For this review, take the finished solid that the model builds, in its own axes (mm). Face numbers are marked on the shaded views. A direction names the side the tool comes from. Round coordinates to 2 decimals unless told otherwise and drop trailing zeros. Write each loop counter-clockwise with the first axis right and the second up, starting at its lowest first coordinate (ties: lowest second). Pieces come first, ordered by that corner, then holes. Notation, with made-up numbers: (3, 27.25) - (55, 27.25) arc R25 ccw to (55, 55.25) - close; hole circle Ø1 at (22, 12). An arc over 180 degrees is marked (long way). One line per item, written item: value. Start each with the question number.
Q1. Mouldability with a two-part tool opening along X and no side actions: class the marked faces 1, 2 and 3 as +X half, -X half, draft (parallel to the pull), parting line (faces both ways), or undercut.
Q2. Clearance check with flat-ended pins moving along their axes: pin 1 Ø1.7 at (x, y) = (-35, -6.5) entering from +Z; pin 2 Ø1.5 at (x, z) = (18.5, 5) entering from +Y; pin 3 Ø3.5 at (x, y) = (14.75, 5) entering from -Z; pin 4 Ø3 at (y, z) = (2.5, 4) entering from +X. State where each tip first meets the part, or that it passes through.
Q3. Add section B-B on x = -9. Write out the cut boundary in (y, z).
Q4. Add section A-A on y = 0. Write out the cut boundary in (x, z).
Q5. For probe 1 along Y at (x, z) = (14.75, 1.95); probe 2 along Y at (x, z) = (-34.75, 1.75); probe 3 along X at (y, z) = (7.5, 5.5), list the stretches that pass through material, from the lowest coordinate up.
Q6. Add section C-C on x = 35. Write out the cut boundary in (y, z), and give its area (3 significant figures).
Q7. Tool access review of the marked faces 4, 5 and 6: name each direction out of +Z, -Z, +X, -X, +Y, -Y from which nothing blocks a thin tool from reaching the whole face with its end or side.
```python
from build123d import *

# Parameters (mm, degrees)
SZKIC1_R                    = 1.55
SZKIC1_R_2                  = 1.45
DODANIE_WYCI_GNI_CIE1_DEPTH = 8
WYTNIJ_WYCI_GNI_CIE1_DEPTH  = 3
ZAOKR_GLENIE1_R             = 4
WYTNIJ_WYCI_GNI_CIE2_DEPTH  = 3.5
SFAZOWANIE1_SIZE            = 0.25
WYTNIJ_WYCI_GNI_CIE3_DEPTH  = 1
WYTNIJ_WYCI_GNI_CIE4_DEPTH  = 3
SZYK_LINIOWY1_COUNT         = 2
SZYK_LINIOWY1_PITCH         = 15


with BuildPart() as part:
    # Szkic1 → Dodanie-wyciągnięcie1 (new body)
    # profile 1 of 17: a face of its own
    with BuildSketch(Plane.XY):
        with BuildLine():
            Line((-30, -5), (-30, 5))
            ThreePointArc((-30, 5), (-34.75, 9.75), (-39.5, 5))
            Line((-39.5, 5), (-39.5, -5))
            ThreePointArc((-39.5, -5), (-34.75, -9.75), (-30, -5))
        make_face()
        with Locations((-34.75, -5)):
            Circle(SZKIC1_R, mode=Mode.SUBTRACT)
        with Locations((-34.75, 5)):
            Circle(SZKIC1_R, mode=Mode.SUBTRACT)
    # profile 2 of 17: a face of its own
    with BuildSketch(Plane.XY):
        with BuildLine():
            Line((-30, -10), (-30, -5))
            ThreePointArc((-30, -5), (-34.75, -9.75), (-39.5, -5))
            ThreePointArc((-39.5, -5), (-36.846817098, -13.293438899), (-29.872582883, -18.506937282))
            ThreePointArc((-29.872582883, -18.506937282), (-32.348896474, -13.420890585), (-27.262849777, -10.944576994))
            Line((-27.262849777, -10.944576994), (-30, -10))
        make_face()
    # profile 3 of 17: a face of its own
    with BuildSketch(Plane.XY):
        with BuildLine():
            Line((4.547807332, -21.922277315), (-27.262849777, -10.944576994))
            ThreePointArc((-27.262849777, -10.944576994), (-32.348896474, -13.420890585), (-29.872582883, -18.506937282))
            Line((-29.872582883, -18.506937282), (5.695133447, -30.781180144))
            ThreePointArc((5.695133447, -30.781180144), (3.398037408, -28.739501506), (3.227247846, -25.670962309))
            Line((3.227247846, -25.670962309), (4.547807332, -21.922277315))
        make_face()
    # profile 4 of 17: a face of its own
    with BuildSketch(Plane.XY):
        with BuildLine():
            Line((7.670780796, -23), (4.547807332, -21.922277315))
            Line((4.547807332, -21.922277315), (3.227247846, -25.670962309))
            ThreePointArc((3.227247846, -25.670962309), (4.688739604, -23.735329208), (7, -23))
            Line((7, -23), (7.670780796, -23))
        make_face()
    # profile 5 of 17: a face of its own
    with BuildSketch(Plane.XY):
        with BuildLine():
            Line((10, -6.445085227), (4.547807332, -21.922277315))
            Line((4.547807332, -21.922277315), (7.670780796, -23))
            Line((7.670780796, -23), (12.650026795, -23))
            Line((12.650026795, -23), (16.842670109, -11.098302851))
            Line((16.842670109, -11.098302851), (14.743601006, -9.74999569))
            ThreePointArc((14.743601006, -9.74999569), (11.798045524, -8.721352546), (10.126086359, -6.087162658))
            Line((10.126086359, -6.087162658), (10, -6.445085227))
        make_face()
    # profile 6 of 17: a face of its own
    with BuildSketch(Plane.XY):
        with BuildLine():
            ThreePointArc((3.227247846, -25.670962309), (3.398037408, -28.739501506), (5.695133447, -30.781180144))
            ThreePointArc((5.695133447, -30.781180144), (6.338456568, -30.944915752), (7, -31))
            ThreePointArc((7, -31), (9.311260396, -30.264670792), (10.772752154, -28.329037691))
            ThreePointArc((10.772752154, -28.329037691), (10.601962592, -25.260498494), (8.304866553, -23.218819856))
            Line((8.304866553, -23.218819856), (7.670780796, -23))
            Line((7.670780796, -23), (7, -23))
            ThreePointArc((7, -23), (4.688739604, -23.735329208), (3.227247846, -25.670962309))
        make_face()
        with Locations((7, -27)):
            Circle(SZKIC1_R_2, mode=Mode.SUBTRACT)
    # profile 7 of 17: a face of its own
    with BuildSketch(Plane.XY):
        with BuildLine():
            Line((10, -5), (10, -6.445085227))
            Line((10, -6.445085227), (10.126086359, -6.087162658))
            ThreePointArc((10.126086359, -6.087162658), (10.03162688, -5.547224911), (10, -5))
        make_face()
    # profile 8 of 17: a face of its own
    with BuildSketch(Plane.XY):
        with BuildLine():
            Line((12.650026795, -23), (7.670780796, -23))
            Line((7.670780796, -23), (8.304866553, -23.218819856))
            ThreePointArc((8.304866553, -23.218819856), (10.601962592, -25.260498494), (10.772752154, -28.329037691))
            Line((10.772752154, -28.329037691), (12.650026795, -23))
        make_face()
    # profile 9 of 17: a face of its own
    with BuildSketch(Plane.XY):
        with BuildLine():
            ThreePointArc((10.772752154, -28.329037691), (9.311260396, -30.264670792), (7, -31))
            Line((7, -31), (49, -31))
            ThreePointArc((49, -31), (47.873511508, -30.838101572), (46.838211374, -30.365511839))
            Line((46.838211374, -30.365511839), (35.371448625, -23))
            Line((35.371448625, -23), (12.650026795, -23))
            Line((12.650026795, -23), (10.772752154, -28.329037691))
        make_face()
    # profile 10 of 17: a face of its own
    with BuildSketch(Plane.XY):
        with BuildLine():
            ThreePointArc((10, -5), (10.03162688, -5.547224911), (10.126086359, -6.087162658))
            Line((10.126086359, -6.087162658), (10.977247846, -3.670962309))
            ThreePointArc((10.977247846, -3.670962309), (13.45169048, -1.216563415), (16.911788626, -1.634488161))
            Line((16.911788626, -1.634488161), (19.5, -3.296988898))
            Line((19.5, -3.296988898), (19.5, 5))
            ThreePointArc((19.5, 5), (14.75, 9.75), (10, 5))
            Line((10, 5), (10, -5))
        make_face()
        with Locations((14.75, 5)):
            Circle(SZKIC1_R, mode=Mode.SUBTRACT)
    # profile 11 of 17: a face of its own
    with BuildSketch(Plane.XY):
        with BuildLine():
            Line((10.977247846, -3.670962309), (10.126086359, -6.087162658))
            ThreePointArc((10.126086359, -6.087162658), (11.798045524, -8.721352546), (14.743601006, -9.74999569))
            Line((14.743601006, -9.74999569), (12.588211374, -8.365511839))
            ThreePointArc((12.588211374, -8.365511839), (10.966563415, -6.29830952), (10.977247846, -3.670962309))
        make_face()
    # profile 12 of 17: a face of its own
    with BuildSketch(Plane.XY):
        Polygon((16.842670109, -11.098302851), (12.650026795, -23), (35.371448625, -23), align=None)
    # profile 13 of 17: a face of its own
    with BuildSketch(Plane.XY):
        with BuildLine():
            ThreePointArc((46.838211374, -30.365511839), (47.873511508, -30.838101572), (49, -31))
            ThreePointArc((49, -31), (52.838101572, -28.126488492), (51.161788626, -23.634488161))
            ThreePointArc((51.161788626, -23.634488161), (50.126488492, -23.161898428), (49, -23))
            Line((49, -23), (35.371448625, -23))
            Line((35.371448625, -23), (46.838211374, -30.365511839))
        make_face()
        with Locations((49, -27)):
            Circle(SZKIC1_R_2, mode=Mode.SUBTRACT)
    # profile 14 of 17: a face of its own
    with BuildSketch(Plane.XY):
        with BuildLine():
            ThreePointArc((16.911788626, -1.634488161), (13.45169048, -1.216563415), (10.977247846, -3.670962309))
            ThreePointArc((10.977247846, -3.670962309), (10.966563415, -6.29830952), (12.588211374, -8.365511839))
            Line((12.588211374, -8.365511839), (14.743601006, -9.74999569))
            ThreePointArc((14.743601006, -9.74999569), (16.291742556, -9.492830944), (17.671590668, -8.745238039))
            Line((17.671590668, -8.745238039), (18.522752154, -6.329037691))
            ThreePointArc((18.522752154, -6.329037691), (18.533436585, -3.70169048), (16.911788626, -1.634488161))
        make_face()
        with Locations((14.75, -5)):
            Circle(SZKIC1_R, mode=Mode.SUBTRACT)
    # profile 15 of 17: a face of its own
    with BuildSketch(Plane.XY):
        with BuildLine():
            ThreePointArc((17.671590668, -8.745238039), (16.291742556, -9.492830944), (14.743601006, -9.74999569))
            Line((14.743601006, -9.74999569), (16.842670109, -11.098302851))
            Line((16.842670109, -11.098302851), (17.671590668, -8.745238039))
        make_face()
    # profile 16 of 17: a face of its own
    with BuildSketch(Plane.XY):
        with BuildLine():
            Line((16.842670109, -11.098302851), (35.371448625, -23))
            Line((35.371448625, -23), (49, -23))
            ThreePointArc((49, -23), (50.126488492, -23.161898428), (51.161788626, -23.634488161))
            Line((51.161788626, -23.634488161), (19.5, -3.296988898))
            Line((19.5, -3.296988898), (19.5, -5))
            ThreePointArc((19.5, -5), (19.018492455, -7.083859919), (17.671590668, -8.745238039))
            Line((17.671590668, -8.745238039), (16.842670109, -11.098302851))
        make_face()
    # profile 17 of 17: a face of its own
    with BuildSketch(Plane.XY):
        with BuildLine():
            Line((19.5, -3.296988898), (16.911788626, -1.634488161))
            ThreePointArc((16.911788626, -1.634488161), (18.533436585, -3.70169048), (18.522752154, -6.329037691))
            Line((18.522752154, -6.329037691), (17.671590668, -8.745238039))
            ThreePointArc((17.671590668, -8.745238039), (19.018492455, -7.083859919), (19.5, -5))
            Line((19.5, -5), (19.5, -3.296988898))
        make_face()
    extrude(amount=DODANIE_WYCI_GNI_CIE1_DEPTH)

    # Szkic2 → Wytnij-wyciągnięcie1 (cut)
    with BuildSketch(Plane(origin=(0, 0, 0), x_dir=(-1, 0, 0), z_dir=(0, 0, -1))):
        Polygon((-45.766838493, -27), (-47.383419246, -24.2), (-50.616580754, -24.2), (-52.233161507, -27), (-50.616580754, -29.8), (-47.383419246, -29.8), align=None)
        Polygon((-10.233161507, -27), (-8.616580754, -29.8), (-5.383419246, -29.8), (-3.766838493, -27), (-5.383419246, -24.2), (-8.616580754, -24.2), align=None)
    extrude(amount=-WYTNIJ_WYCI_GNI_CIE1_DEPTH, mode=Mode.SUBTRACT)

    # Zaokrąglenie1
    zaokr_glenie1_edges = [part.edges().sort_by_distance(p)[0] for p in [
        (4.547807332, -21.922277315, 4),
        (10, -6.445085227, 4),
        (19.5, -3.296988898, 4),
    ]]
    fillet(zaokr_glenie1_edges, radius=ZAOKR_GLENIE1_R)

    # Szkic3 → Wytnij-wyciągnięcie2 (cut)
    with BuildSketch(Plane.XY.offset(8)):
        Polygon((-34.75, 1.766838493), (-31.95, 3.383419246), (-31.95, 6.616580754), (-34.75, 8.233161507), (-37.55, 6.616580754), (-37.55, 3.383419246), align=None)
        Polygon((-34.75, -8.233161507), (-31.95, -6.616580754), (-31.95, -3.383419246), (-34.75, -1.766838493), (-37.55, -3.383419246), (-37.55, -6.616580754), align=None)
        Polygon((14.75, 1.766838493), (17.55, 3.383419246), (17.55, 6.616580754), (14.75, 8.233161507), (11.95, 6.616580754), (11.95, 3.383419246), align=None)
        Polygon((14.75, -8.233161507), (17.55, -6.616580754), (17.55, -3.383419246), (14.75, -1.766838493), (11.95, -3.383419246), (11.95, -6.616580754), align=None)
    extrude(amount=-WYTNIJ_WYCI_GNI_CIE2_DEPTH, mode=Mode.SUBTRACT)

    # Sfazowanie1
    sfazowanie1_edges = [part.edges().sort_by_distance(p)[0] for p in [
        (36.25, -14.056112985, 8),
        (7.820559487, -12.631884103, 0),
        (7.820559487, -12.631884103, 8),
        (-14.604625944, -15.312867387, 0),
        (-14.604625944, -15.312867387, 8),
        (19.9895047, -3.029625968, 0),
        (19.9895047, -3.029625968, 8),
        (9.942778755, -6.435301151, 0),
        (9.942778755, -6.435301151, 8),
        (3.835116171, -20.446517222, 0),
        (3.835116171, -20.446517222, 8),
        (19.5, 1.943887015, 8),
        (14.75, 9.75, 8),
        (10, -0.380569097, 8),
        (52.838101572, -28.126488492, 0),
        (28, -31, 0),
        (6.338456568, -30.944915752, 0),
        (-12.088724718, -24.644058713, 0),
        (-36.846817098, -13.293438899, 0),
        (-39.5, 0, 0),
        (-34.75, 9.75, 0),
        (-30, -2.5, 0),
        (10, -0.380569097, 0),
        (14.75, 9.75, 0),
        (19.5, 1.943887015, 0),
        (36.25, -14.056112985, 0),
        (-30, -2.5, 8),
        (-34.75, 9.75, 8),
        (-39.5, 0, 8),
        (-36.846817098, -13.293438899, 8),
        (-12.088724718, -24.644058713, 8),
        (6.338456568, -30.944915752, 8),
        (28, -31, 8),
        (52.838101572, -28.126488492, 8),
    ]]
    chamfer(sfazowanie1_edges, length=SFAZOWANIE1_SIZE)

    # Szkic4 → Wytnij-wyciągnięcie3 (cut)
    with BuildSketch(Plane(origin=(0, 0, 0), x_dir=(-1, 0, 0), z_dir=(0, 0, -1))):
        Polygon((-40.766838493, -25.5), (-40.766838493, -28.5), (-37.058739249, -27), align=None)
    extrude(amount=-WYTNIJ_WYCI_GNI_CIE3_DEPTH, mode=Mode.SUBTRACT)

    # Szkic5 → Wytnij-wyciągnięcie4 (cut)
    with BuildSketch(Plane(origin=(42.74800903, -18.230016596, 0.25), x_dir=(0, 0, 1), z_dir=(-0.841377959640588, 0.5404471565574577, 0))):
        with BuildLine():
            Line((2.25, 0), (3.75, 0))
            ThreePointArc((3.75, 0), (2.578427125, -2.828427125), (-0.25, -4))
            Line((-0.25, -4), (-0.25, -2.5))
            ThreePointArc((-0.25, -2.5), (1.517766953, -1.767766953), (2.25, 0))
        make_face()
    wytnij_wyci_gni_cie4 = extrude(amount=WYTNIJ_WYCI_GNI_CIE4_DEPTH, mode=Mode.SUBTRACT)

    # Szyk liniowy1: Wytnij-wyciągnięcie4 ×2
    with Locations(*[Vector(-0.8413779596405879, 0.5404471565574578, 0) * (i * SZYK_LINIOWY1_PITCH) for i in range(1, SZYK_LINIOWY1_COUNT)]):
        add(wytnij_wyci_gni_cie4, mode=Mode.SUBTRACT)


solid = part.part
```
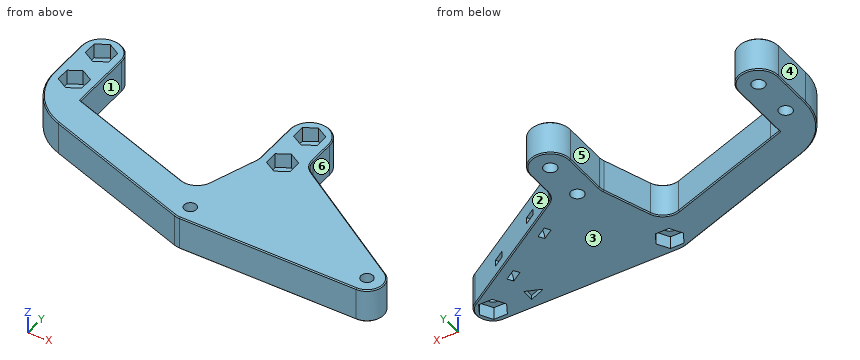
Result set:
1. face 1: undercut
1. face 2: +X half
1. face 3: draft
2. pin 1: stops at z = 4.5
2. pin 2: stops at y = 8.68
2. pin 3: stops at z = 0
2. pin 4: stops at x = 19.5
3. outline: (-25.71, 0.25) - (-25.45, 0) - (-17.51, 0) - (-17.25, 0.25) - (-17.25, 7.75) - (-17.51, 8) - (-25.45, 8) - (-25.71, 7.75) - close
4. outline: (-39.5, 0.25) - (-39.25, 0) - (-30.25, 0) - (-30, 0.25) - (-30, 7.75) - (-30.25, 8) - (-39.25, 8) - (-39.5, 7.75) - close; (10, 0.25) - (10.25, 0) - (19.25, 0) - (19.5, 0.25) - (19.5, 7.75) - (19.25, 8) - (10.25, 8) - (10, 7.75) - close
5. probe 1: y = -31 to -6.55, -3.45 to 3.45, 6.55 to 9.75
5. probe 2: y = -15.64 to -6.55, -3.45 to 3.45, 6.55 to 9.75
5. probe 3: x = -38.79 to -36.02, -33.48 to -30.71, 10.71 to 13.48, 16.02 to 18.79
6. outline: (-31, 0.25) - (-30.75, 0) - (-13.55, 0) - (-13.25, 0.25) - (-13.25, 7.75) - (-13.55, 8) - (-30.75, 8) - (-31, 7.75) - close
6. area: 142 mm^2
7. face 4: +Z, -Z, -X, +Y, -Y
7. face 5: +Z, -Z, +Y
7. face 6: +Z, -Z, +X, +Y
